from build123d import *

# Parameters (mm, degrees)
SZKIC1_W                               = 35
SZKIC1_H                               = 5
DODANIE_WYCI_GNI_CIE1_DEPTH            = 45
DODANIE_WYCI_GNI_CIE2_START            = 10
SZKIC2_R                               = 12
SZKIC2_R_2                             = 4.25
DODANIE_WYCI_GNI_CIE2_DEPTH            = 25
DODANIE_WYCI_GNI_CIE3_START            = -14
DODANIE_WYCI_GNI_CIE3_DEPTH            = 7
DODANIE_WYCI_GNI_CIE4_START            = -19
DODANIE_WYCI_GNI_CIE4_DEPTH            = 7
WYTNIJ_WYCI_GNI_CIE1_REACH             = 61.634
SZKIC5_R                               = 2
WYTNIJ_WYCI_GNI_CIE2_REACH             = 51.308
SZKIC10_R                              = 1.5
WYTNIJ_WYCI_GNI_CIE2_DIRECTION_2_DEPTH = 3
SZYK_KO_OWY1_COUNT                     = 4
SFAZOWANIE1_SIZE                       = 1
SFAZOWANIE1_SIZE2                      = 0.624869352


with BuildPart() as part:
    # Szkic1 → Dodanie-wyci_gni_cie1 (new body)
    with BuildSketch(Plane(origin=(0, 0, 0), x_dir=(1, 0, 0), z_dir=(0, 1, 0))):
        with Locations((0, 2.5)):
            Rectangle(SZKIC1_W, SZKIC1_H)
    extrude(amount=DODANIE_WYCI_GNI_CIE1_DEPTH)



with BuildPart() as body_2:
    # Szkic2 → Dodanie-wyci_gni_cie2 (new body)
    with BuildSketch(Plane(origin=(0, 0, 0), x_dir=(1, 0, 0), z_dir=(0, 1, 0)).offset(DODANIE_WYCI_GNI_CIE2_START)):
        with Locations(Location((0, -18, 0), (0, 0, 270))):
            Circle(SZKIC2_R)
        with Locations(Location((0, -18, 0), (0, 0, 270))):
            Circle(SZKIC2_R_2, mode=Mode.SUBTRACT)
    extrude(amount=DODANIE_WYCI_GNI_CIE2_DEPTH)


with BuildPart() as part_1:
    add(part.part)

    add(body_2.part)  # Dodanie-wyci_gni_cie3 merges body 2
    # Szkic3 → Dodanie-wyci_gni_cie3 (add)
    with BuildSketch(Plane.ZY.offset(17.5).offset(DODANIE_WYCI_GNI_CIE3_START)):
        Polygon((0, 0), (0, 45), (9.234999726, 35), (9.234999726, 10), align=None)
    extrude(amount=-DODANIE_WYCI_GNI_CIE3_DEPTH)

    # Szkic4 → Dodanie-wyci_gni_cie4 (add)
    with BuildSketch(Plane.XZ.offset(DODANIE_WYCI_GNI_CIE4_START)):
        Polygon((-17.5, 0), (-12, 18), (0, 9.234999726), (12, 18), (17.5, 0), align=None)
    extrude(amount=-DODANIE_WYCI_GNI_CIE4_DEPTH)

    # Szkic5 → Wytnij-wyci_gni_cie1 (cut, up to next)
    with BuildSketch(Plane(origin=(0, 0, -5), x_dir=(-1, 0, 0), z_dir=(0, 0, -1)), mode=Mode.PRIVATE) as wytnij_wyci_gni_cie1_sk1:
        with Locations((-12.5, 40)):
            Circle(SZKIC5_R)
    wytnij_wyci_gni_cie1_tool1 = extrude(wytnij_wyci_gni_cie1_sk1.sketch, amount=-WYTNIJ_WYCI_GNI_CIE1_REACH, mode=Mode.PRIVATE) & part_1.part
    # Szkic5 → Wytnij-wyci_gni_cie1 (cut, up to next)
    with BuildSketch(Plane(origin=(0, 0, -5), x_dir=(-1, 0, 0), z_dir=(0, 0, -1)), mode=Mode.PRIVATE) as wytnij_wyci_gni_cie1_sk2:
        with Locations((12.5, 40)):
            Circle(SZKIC5_R)
    wytnij_wyci_gni_cie1_tool2 = extrude(wytnij_wyci_gni_cie1_sk2.sketch, amount=-WYTNIJ_WYCI_GNI_CIE1_REACH, mode=Mode.PRIVATE) & part_1.part
    # Szkic5 → Wytnij-wyci_gni_cie1 (cut, up to next)
    with BuildSketch(Plane(origin=(0, 0, -5), x_dir=(-1, 0, 0), z_dir=(0, 0, -1)), mode=Mode.PRIVATE) as wytnij_wyci_gni_cie1_sk3:
        with Locations((12.5, 5)):
            Circle(SZKIC5_R)
    wytnij_wyci_gni_cie1_tool3 = extrude(wytnij_wyci_gni_cie1_sk3.sketch, amount=-WYTNIJ_WYCI_GNI_CIE1_REACH, mode=Mode.PRIVATE) & part_1.part
    # Szkic5 → Wytnij-wyci_gni_cie1 (cut, up to next)
    with BuildSketch(Plane(origin=(0, 0, -5), x_dir=(-1, 0, 0), z_dir=(0, 0, -1)), mode=Mode.PRIVATE) as wytnij_wyci_gni_cie1_sk4:
        with Locations((-12.5, 5)):
            Circle(SZKIC5_R)
    wytnij_wyci_gni_cie1_tool4 = extrude(wytnij_wyci_gni_cie1_sk4.sketch, amount=-WYTNIJ_WYCI_GNI_CIE1_REACH, mode=Mode.PRIVATE) & part_1.part
    add(wytnij_wyci_gni_cie1_tool1.solids().sort_by_distance((12.5, 40, -5))[0], mode=Mode.SUBTRACT)
    add(wytnij_wyci_gni_cie1_tool2.solids().sort_by_distance((-12.5, 40, -5))[0], mode=Mode.SUBTRACT)
    add(wytnij_wyci_gni_cie1_tool3.solids().sort_by_distance((-12.5, 5, -5))[0], mode=Mode.SUBTRACT)
    add(wytnij_wyci_gni_cie1_tool4.solids().sort_by_distance((12.5, 5, -5))[0], mode=Mode.SUBTRACT)

    # Szkic10 → Wytnij-wyci_gni_cie2 (cut, up to next)
    with BuildSketch(Plane(origin=(0, 10, 0), x_dir=(-1, 0, 0), z_dir=(0, -1, 0)), mode=Mode.PRIVATE) as wytnij_wyci_gni_cie2_sk1:
        with Locations(Location((-8, -18, 0), (0, 0, 270))):
            Circle(SZKIC10_R)
    wytnij_wyci_gni_cie2_tool1 = extrude(wytnij_wyci_gni_cie2_sk1.sketch, amount=-WYTNIJ_WYCI_GNI_CIE2_REACH, mode=Mode.PRIVATE) & part_1.part
    wytnij_wyci_gni_cie2 = wytnij_wyci_gni_cie2_tool1.solids().sort_by_distance((8, 10, 18))[0]
    add(wytnij_wyci_gni_cie2, mode=Mode.SUBTRACT)

    # Szkic10 → Wytnij-wyci_gni_cie2 direction 2 (cut)
    with BuildSketch(Plane(origin=(0, 10, 0), x_dir=(-1, 0, 0), z_dir=(0, -1, 0))):
        with Locations(Location((-8, -18, 0), (0, 0, 270))):
            Circle(SZKIC10_R)
    wytnij_wyci_gni_cie2_direction_2 = extrude(amount=WYTNIJ_WYCI_GNI_CIE2_DIRECTION_2_DEPTH, mode=Mode.SUBTRACT)

    # Szyk ko_owy1: Wytnij-wyci_gni_cie2, Wytnij-wyci_gni_cie2 direction 2; each copy of Wytnij-wyci_gni_cie2 runs up to whatever stops it at its own place
    szyk_ko_owy1_before = part_1.part  # the part as the pattern finds it: every copy runs up to it
    szyk_ko_owy1_wytnij_wyci_gni_cie2_long = extrude(wytnij_wyci_gni_cie2_sk1.sketch, amount=-WYTNIJ_WYCI_GNI_CIE2_REACH, mode=Mode.PRIVATE)
    szyk_ko_owy1_wytnij_wyci_gni_cie2_tool1 = szyk_ko_owy1_wytnij_wyci_gni_cie2_long.rotate(Axis((0, 0, 18), (0, 1, 0)), 1 * 360 / SZYK_KO_OWY1_COUNT) & szyk_ko_owy1_before
    add(szyk_ko_owy1_wytnij_wyci_gni_cie2_tool1.solids().sort_by_distance((0, 10, 10))[0], mode=Mode.SUBTRACT)
    szyk_ko_owy1_wytnij_wyci_gni_cie2_tool2 = szyk_ko_owy1_wytnij_wyci_gni_cie2_long.rotate(Axis((0, 0, 18), (0, 1, 0)), 2 * 360 / SZYK_KO_OWY1_COUNT) & szyk_ko_owy1_before
    add(szyk_ko_owy1_wytnij_wyci_gni_cie2_tool2.solids().sort_by_distance((-8, 10, 18))[0], mode=Mode.SUBTRACT)
    szyk_ko_owy1_wytnij_wyci_gni_cie2_tool3 = szyk_ko_owy1_wytnij_wyci_gni_cie2_long.rotate(Axis((0, 0, 18), (0, 1, 0)), 3 * 360 / SZYK_KO_OWY1_COUNT) & szyk_ko_owy1_before
    add(szyk_ko_owy1_wytnij_wyci_gni_cie2_tool3.solids().sort_by_distance((0, 10, 26))[0], mode=Mode.SUBTRACT)
    add(wytnij_wyci_gni_cie2_direction_2.rotate(Axis((0, 0, 18), (0, 1, 0)), 1 * 360 / SZYK_KO_OWY1_COUNT), mode=Mode.SUBTRACT)
    add(wytnij_wyci_gni_cie2_direction_2.rotate(Axis((0, 0, 18), (0, 1, 0)), 2 * 360 / SZYK_KO_OWY1_COUNT), mode=Mode.SUBTRACT)
    add(wytnij_wyci_gni_cie2_direction_2.rotate(Axis((0, 0, 18), (0, 1, 0)), 3 * 360 / SZYK_KO_OWY1_COUNT), mode=Mode.SUBTRACT)

    # Sfazowanie1
    sfazowanie1_edges = [part_1.edges().sort_by_distance(p)[0] for p in [
        (0, 10, 13.75),
    ]]
    sfazowanie1_side = [part_1.faces().sort_by_distance(p)[0] for p in [
        (0, 22.5, 13.75),
    ]]
    chamfer(sfazowanie1_edges, length=SFAZOWANIE1_SIZE, length2=SFAZOWANIE1_SIZE2, reference=sfazowanie1_side[0])


solid = part_1.part
CAD build for the part. Positions are in the model's coordinates, mm. A direction names the side the tool comes from. Coordinates: 2 decimals unless noted, no trailing zeros. Order: outer loops, then holes, each group sorted by start corner. A loop starts at its lowest first (then second) coordinate and runs counter-clockwise, first axis right, second up.
Item 1: Band-saw the part on D-D on x = -8. List the corners of the cut face in (y, z).
Check sheet entries:
outline: (0, -5) - (45, -5) - (45, 0) - (26, 0) - (26, 9.06) - (35, 9.06) - (35, 16.5) - (10, 16.5) - (10, 9.06) - (19, 9.06) - (19, 0) - (0, 0) - close; (10, 19.5) - (35, 19.5) - (35, 26.94) - (10, 26.94) - close
Item 2: Band-saw the part on B-B on x = 13. List the corners of the cut face in (y, z).
Check sheet entries:
outline: (0, -5) - (3.06, -5) - (3.06, 0) - (0, 0) - close; (6.94, -5) - (38.06, -5) - (38.06, 0) - (26, 0) - (26, 14.73) - (19, 14.73) - (19, 0) - (6.94, 0) - close; (41.94, -5) - (45, -5) - (45, 0) - (41.94, 0) - close
Item 3: Band-saw the part on C-C on y = 40. List the corners of the cut face in (x, z).
Check sheet entries:
outline: (-17.5, -5) - (-14.5, -5) - (-14.5, 0) - (-17.5, 0) - close; (-10.5, -5) - (10.5, -5) - (10.5, 0) - (3.5, 0) - (3.5, 4.62) - (-3.5, 4.62) - (-3.5, 0) - (-10.5, 0) - close; (14.5, -5) - (17.5, -5) - (17.5, 0) - (14.5, 0) - close
Item 4: Two-plate mould, pull along Y, no slides. Class faces 1 (the face through (-10, 19, 5)), 2 (the face through (14.498, 5.088, -2.535)), 3 (the face through (14.71, 22.45, 9.13)): +Y half, -Y half, draft (parallel to the pull), parting line (faces both ways), or undercut.
Check sheet entries:
face 1: -Y half
face 2: undercut
face 3: draft
Item 5: 3-axis set-ups, long thin cutter, end or side, ignore diameter. For faces 4 (the face through (-11, 9, 0)), 5 (the face through (-3.5, 34, 3)), 6 (the face through (0, 22, 30)), 7 (the face through (11, 19, 5)): which of +Z, -Z, +X, -X, +Y, -Y reach the whole face in a straight line?
Check sheet entries:
face 4: -X, -Y
face 5: -X, +Y
face 6: none
face 7: +X, -Y
Item 6: Pin check, flat tips, straight feed: pin 1 Ø12 at (x, y) = (8, 29.5) entering from +Z; pin 2 Ø12 at (y, z) = (6.5, 4) entering from +X; pin 3 Ø4 at (x, z) = (-8, 18) entering from +Y; pin 4 Ø4 at (x, y) = (-7.5, 14.5) entering from +Z. Stop position of each tip, or through.
Check sheet entries:
pin 1: stops at z = 29.83
pin 2: stops at x = 17.5
pin 3: stops at y = 35
pin 4: stops at z = 28.67
Item 7: Band-saw the part on A-A on z = 26. List the corners of the cut face in (x, y).
Check sheet entries:
outline: (-8.94, 10) - (-1.5, 10) - (-1.5, 35) - (-8.94, 35) - close; (1.5, 10) - (8.94, 10) - (8.94, 35) - (1.5, 35) - close
Item 8: Drill centre lines: L1, parallel to X at y = 18, z = 18; L2, parallel to Y at x = -12.5, z = -2.95; L3, parallel to Z at x = -0.5, y = 19. Where is each one in solid material? Low to high.
Check sheet entries:
L1: x = -12 to -9.5, -6.5 to -4.25, 4.25 to 6.5, 9.5 to 12
L2: y = 0 to 3, 7 to 38, 42 to 45
L3: z = -5 to 8.59, 11.41 to 13.78, 22.22 to 24.59, 27.41 to 29.99
